Geometry check sheet. Reference: the model listing, model coordinates, mm. Round coordinates to 2 decimals unless told otherwise and drop trailing zeros. Write each loop counter-clockwise with the first axis right and the second up, starting at its lowest first coordinate (ties: lowest second). Pieces come first, ordered by that corner, then holes. Notation, with made-up numbers: M 37,26 L 62,26 A29 cw 62,55 Z; hole C 13.5,-22 d4. An arc over 180 degrees is marked long. Answer as CSV lines item,"result". Start each with the question number.
```python
from build123d import *

# Parameters (mm, degrees)
SKETCH1_W           = 50
SKETCH1_H           = 30
BOSS_EXTRUDE1_DEPTH = 5
CHAMFER1_SIZE       = 5


with BuildPart() as part:
    # Sketch1 → Boss-Extrude1 (new body)
    with BuildSketch(Plane(origin=(0, 0, 0), x_dir=(1, 0, 0), z_dir=(0, 1, 0))):
        Rectangle(SKETCH1_W, SKETCH1_H)
    extrude(amount=BOSS_EXTRUDE1_DEPTH)

    # Chamfer1
    chamfer1_edges = [part.edges().sort_by_distance(p)[0] for p in [
        (0, 0, 15),
    ]]
    chamfer(chamfer1_edges, length=CHAMFER1_SIZE - 0.0001)  # a hair under: the kernel refuses the full size


solid = part.part
```
1) Scan lines: line 1 (Z direction, x = 0, y = 1.6); line 2 (Z direction, x = 9.5, y = 3). Record each from-to range of solid material in increasing order. Write a range as from..to.
2) Mould release check, pull along Z, two halves, no side actions. Record for faces 1 (the flat face through (0, 2, -15)), 2 (the flat face through (0, 0, -3)), 3 (the flat face through (0, 2, 12)): released by +Z, released by -Z, zero draft, split by the parting line, or undercut.
3) Section check C-C, the plane y = 1.4. Record the cut outline in (x, z).
4) Section check B-B, the plane y = 4.05. Record the cut outline in (x, z).
Results:
1,line 1,"z = -15..11.6"
1,line 2,"z = -15..13"
2,face 1,"released by -Z"
2,face 2,"zero draft"
2,face 3,"released by +Z"
3,outline,"M -25,-15 L 25,-15 L 25,11.4 L -25,11.4 Z"
4,outline,"M -25,-15 L 25,-15 L 25,14.05 L -25,14.05 Z"
